```python
from build123d import *

# Parameters (mm, degrees)
SKETCH1_W                       = 75
SKETCH1_H                       = 24
BOSS_EXTRUDE1_DEPTH             = 24
SKETCH2_W                       = 20
SKETCH2_H                       = 12
CUT_EXTRUDE1_DEPTH              = 24
FILLET1_START                   = -1
FILLET1_DEPTH                   = 26
FILLET1_2_DEPTH                 = 24
F_8_0MM_DOWEL_HOLE1_D           = 8
F_8_0MM_DOWEL_HOLE1_DEPTH       = 15
F_8_0MM_DOWEL_HOLE1_CSINK_D     = 8.05
F_8_0MM_DOWEL_HOLE1_CSINK_ANGLE = 90
F_8_0MM_DOWEL_HOLE1_TIP         = 2.403442476
M3X0_5_TAPPED_HOLE1_D           = 2.5
M3X0_5_TAPPED_HOLE1_DEPTH       = 7.5
M3X0_5_TAPPED_HOLE1_CSINK_D     = 3.05
M3X0_5_TAPPED_HOLE1_CSINK_ANGLE = 90
M3X0_5_TAPPED_HOLE1_TIP         = 0.751075774
BOSS_EXTRUDE2_DEPTH             = 24
FILLET2_R                       = 0.25


with BuildPart() as part:
    # Sketch1 → Boss-Extrude1 (new body)
    with BuildSketch(Plane(origin=(0, 0, 0), x_dir=(0, 0, -1), z_dir=(1, 0, 0))):
        Rectangle(SKETCH1_W, SKETCH1_H)
    extrude(amount=BOSS_EXTRUDE1_DEPTH)

    # Sketch2 → Cut-Extrude1 (cut)
    with BuildSketch(Plane(origin=(24, 0, 0), x_dir=(0, 0, -1), z_dir=(1, 0, 0))):
        with Locations((-27.5, 6)):
            Rectangle(SKETCH2_W, SKETCH2_H)
    cut_extrude1 = extrude(amount=-CUT_EXTRUDE1_DEPTH, mode=Mode.SUBTRACT)

    # Fillet1: read off the stored shape, not the designer's step
    # Fillet1 outline → Fillet1 (cut)
    with BuildSketch(Plane.YZ.offset(FILLET1_START)):
        with BuildLine():
            Line((12, 17.5), (6, 17.5))
            ThreePointArc((6, 17.5), (10.242640687, 15.742640687), (12, 11.5))
            Line((12, 11.5), (12, 17.5))
        make_face()
    fillet1 = extrude(amount=FILLET1_DEPTH, mode=Mode.SUBTRACT)

    # Fillet1 2 outline → Fillet1 2 (add)
    with BuildSketch(Plane.YZ):
        with BuildLine():
            Line((0, 17.5), (6, 17.5))
            ThreePointArc((6, 17.5), (1.757359313, 19.257359313), (0, 23.5))
            Line((0, 23.5), (0, 17.5))
        make_face()
    fillet1_2 = extrude(amount=FILLET1_2_DEPTH)

    # Mirror1: Cut-Extrude1, Fillet1, Fillet1 2 across plane
    add(cut_extrude1.mirror(Plane.XY), mode=Mode.SUBTRACT)
    add(fillet1.mirror(Plane.XY), mode=Mode.SUBTRACT)
    add(fillet1_2.mirror(Plane.XY))

    # Ø8.0mm Dowel Hole1
    with Locations(Plane(origin=(24, 0, 0), x_dir=(0, 0, -1), z_dir=(1, 0, 0))):
        with Locations((0, 0)):
            CounterSinkHole(F_8_0MM_DOWEL_HOLE1_D / 2, F_8_0MM_DOWEL_HOLE1_CSINK_D / 2, depth=F_8_0MM_DOWEL_HOLE1_DEPTH, counter_sink_angle=F_8_0MM_DOWEL_HOLE1_CSINK_ANGLE)
            with Locations((0, 0, -(F_8_0MM_DOWEL_HOLE1_DEPTH + F_8_0MM_DOWEL_HOLE1_TIP / 2))):  # 118° drill point
                Cone(0, F_8_0MM_DOWEL_HOLE1_D / 2, F_8_0MM_DOWEL_HOLE1_TIP, mode=Mode.SUBTRACT)

    # M3x0.5 Tapped Hole1
    with Locations(Plane(origin=(24, 0, 0), x_dir=(0, 0, -1), z_dir=(1, 0, 0))):
        with Locations((-5.656854249, 5.656854249), (5.656854249, 5.656854249), (5.656854249, -5.656854249), (-5.656854249, -5.656854249)):
            CounterSinkHole(M3X0_5_TAPPED_HOLE1_D / 2, M3X0_5_TAPPED_HOLE1_CSINK_D / 2, depth=M3X0_5_TAPPED_HOLE1_DEPTH, counter_sink_angle=M3X0_5_TAPPED_HOLE1_CSINK_ANGLE)
            with Locations((0, 0, -(M3X0_5_TAPPED_HOLE1_DEPTH + M3X0_5_TAPPED_HOLE1_TIP / 2))):  # 118° drill point
                Cone(0, M3X0_5_TAPPED_HOLE1_D / 2, M3X0_5_TAPPED_HOLE1_TIP, mode=Mode.SUBTRACT)

    # Sketch12 → Boss-Extrude2 (add)
    with BuildSketch(Plane(origin=(24, 0, 0), x_dir=(0, 0, -1), z_dir=(1, 0, 0))):
        Polygon((-18, -24), (18, -24), (11.07179677, -12), (-11.07179677, -12), align=None)
    extrude(amount=-BOSS_EXTRUDE2_DEPTH)

    # Fillet2
    fillet2_edges = [part.edges().sort_by_distance(p)[0] for p in [
        (12, -12, 11.07179677),
        (12, -24, 18),
        (12, -24, -18),
        (12, -12, -11.07179677),
    ]]
    fillet(fillet2_edges, radius=FILLET2_R)


solid = part.part
```
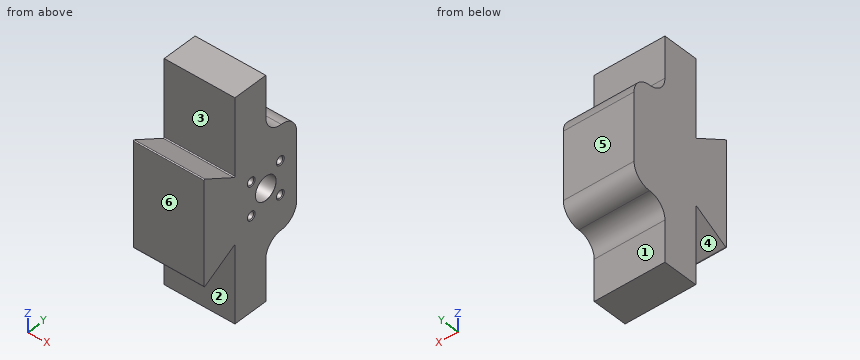
Check sheet for the modelled part. Datum: model origin and axes. Units: mm. Face numbers are marked on the shaded views. A direction names the side the tool comes from. Coordinates: 2 decimals unless noted, no trailing zeros. Order: outer loops, then holes, each group sorted by start corner. A loop starts at its lowest first (then second) coordinate and runs counter-clockwise, first axis right, second up. Notation, with made-up numbers: M 34.25,19.5 L 54.25,19.5 A17 cw 54.25,31.5 Z; hole C 5,67.25 d9. An arc over 180 degrees is marked long. One line per question, with ' | ' between items. Start each with the question number.
Item 1: Access from +Z, -Z, +X, -X, +Y, -Y to the whole of each face (thin tool, end or side, straight path). Record for the marked faces 1, 2 and 3.
Item 2: Sectioned sample at A-A on z = -13. Record the cut outline in (x, y).
Item 3: Mould release check, pull along Y, two halves, no side actions. Record for the marked faces 4, 5 and 6: pulls with the +Y half, pulls with the -Y half, needs draft (parallel to the pull), parting line crosses it, or undercut.
Item 4: Sectioned sample at D-D on z = 25.5. Record the cut outline in (x, y).
Item 5: Gauge pin test, flat ends, axial feed: P1, Ø2, axis at y = 5.66, z = -5.66, coming from the +X side; P2, Ø12, axis at x = 9.5, z = -25, coming from the -Y side; P3, Ø7, axis at y = 0, z = 0, coming from the +X side. Record the tip position at first contact, or that the pin passes through.
Item 6: Material ranges on line 1 (Z direction, x = 19.75, y = 6); line 2 (Z direction, x = 20, y = 5); line 3 (Y direction, x = 16, z = 0), recorded low to high.
Answer below:
1) face 1: -Z, +X, -X, +Y | face 2: -Z, +X, -X | face 3: +Z, +X, -X
2) outline: M 0,-24 L 24,-24 L 24,-15.34 L 0,-15.34 Z; M 0,-12 L 24,-12 L 24,11.81 L 0,11.81 Z
3) face 4: undercut | face 5: pulls with the +Y half | face 6: pulls with the -Y half
4) outline: M 0,-12 L 24,-12 L 24,0 L 0,0 Z
5) P1: stops at x = 16.35 | P2: stops at y = -12 | P3: stops at x = 8.7
6) line 1: z = -17.5 to -6.86, -4.45 to 4.45, 6.86 to 17.5 | line 2: z = -17.58 to -6.72, -4.59 to 4.59, 6.72 to 17.58 | line 3: y = -24 to -4, 4 to 12
